from build123d import *

# Parameters (mm, degrees)
SKETCH7_W               = 50.8
SKETCH7_H               = 49.5808
BASE_FLANGE1_DEPTH      = 3
F_10_CLEARANCE_HOLE1_D  = 5
EDGE_FLANGE1_DEPTH      = 50.8
EDGE_FLANGE1_START      = 3
EDGE_FLANGE1_PROFILE_R  = 2.5
EDGE_FLANGE1_FLAT_DEPTH = 3
EDGE_FLANGE2_DEPTH      = 50.8
EDGE_FLANGE2_START      = 3
EDGE_FLANGE2_PROFILE_R  = 2.5
EDGE_FLANGE2_FLAT_DEPTH = 3


# Sheet-metal steps are written as plain solids
with BuildPart() as part:
    # Sketch7 → Base-Flange1 (new body)
    with BuildSketch(Plane(origin=(0, 0, 0), x_dir=(0, -1, 0), z_dir=(-1, 0, 0))):
        with Locations((-25.4, -28.4)):
            Rectangle(SKETCH7_W, SKETCH7_H)
    extrude(amount=-BASE_FLANGE1_DEPTH)

    # #10 Clearance Hole1 (through all)
    with Locations(Plane(origin=(3, 0, 0), x_dir=(0, 0, -1), z_dir=(1, 0, 0))):
        with Locations((41.1, 12.7), (41.1, 25.4), (28.4, 25.4), (28.4, 12.7), (15.7, 12.7), (15.7, 25.4), (15.7, 38.1), (28.4, 38.1), (41.1, 38.1)):
            Hole(F_10_CLEARANCE_HOLE1_D / 2)

    # Edge-Flange1 bend section (across the edge) → Edge-Flange1 (add)
    with BuildSketch(Plane(origin=(3, 0, -53.8), x_dir=(0, 0, 1), z_dir=(0, 1, 0))):
        with BuildLine():
            Line((-3, 0.6096), (0, 0.6096))
            ThreePointArc((0, 0.6096), (0.178547706, 0.178547706), (0.6096, 0))
            Line((0.6096, 0), (0.6096, -3))
            ThreePointArc((0.6096, -3), (-1.942772637, -1.942772637), (-3, 0.6096))
        make_face()
    extrude(amount=EDGE_FLANGE1_DEPTH)

    # Edge-Flange1 profile (on flange) → Edge-Flange1 flat (add)
    with BuildSketch(Plane(origin=(3, 0, -53.8), x_dir=(0, 1, 0), z_dir=(0, 0, -1)).offset(EDGE_FLANGE1_START)):
        Polygon((0, 0.6096), (50.8, 0.6096), (50.8, 3.35), (66.675, 3.35), (73.025, 9.7), (73.025, 47.8), (66.675, 54.15), (50.8, 54.15), (0, 9.7), align=None)
        with Locations((63.5, 9.7)):
            Circle(EDGE_FLANGE1_PROFILE_R, mode=Mode.SUBTRACT)
        with Locations((63.5, 22.4)):
            Circle(EDGE_FLANGE1_PROFILE_R, mode=Mode.SUBTRACT)
        with Locations((63.5, 35.1)):
            Circle(EDGE_FLANGE1_PROFILE_R, mode=Mode.SUBTRACT)
        with Locations((63.5, 47.8)):
            Circle(EDGE_FLANGE1_PROFILE_R, mode=Mode.SUBTRACT)
    extrude(amount=-EDGE_FLANGE1_FLAT_DEPTH)

    # Edge-Flange2 bend section (across the edge) → Edge-Flange2 (add)
    with BuildSketch(Plane(origin=(3, 50.8, -3), x_dir=(0, 0, -1), z_dir=(0, -1, 0))):
        with BuildLine():
            Line((-3, 0.6096), (0, 0.6096))
            ThreePointArc((0, 0.6096), (0.178547706, 0.178547706), (0.6096, 0))
            Line((0.6096, 0), (0.6096, -3))
            ThreePointArc((0.6096, -3), (-1.942772637, -1.942772637), (-3, 0.6096))
        make_face()
    extrude(amount=EDGE_FLANGE2_DEPTH)

    # Edge-Flange2 profile (on flange) → Edge-Flange2 flat (add)
    with BuildSketch(Plane(origin=(3, 0, -3), x_dir=(0, -1, 0), z_dir=(0, 0, 1)).offset(EDGE_FLANGE2_START)):
        Polygon((0, 0.6096), (0, 9.7), (-50.8, 54.15), (-66.675, 54.15), (-73.025, 47.8), (-73.025, 9.7), (-66.675, 3.35), (-50.8, 3.35), (-50.8, 0.6096), align=None)
        with Locations((-63.5, 9.7)):
            Circle(EDGE_FLANGE2_PROFILE_R, mode=Mode.SUBTRACT)
        with Locations((-63.5, 22.4)):
            Circle(EDGE_FLANGE2_PROFILE_R, mode=Mode.SUBTRACT)
        with Locations((-63.5, 35.1)):
            Circle(EDGE_FLANGE2_PROFILE_R, mode=Mode.SUBTRACT)
        with Locations((-63.5, 47.8)):
            Circle(EDGE_FLANGE2_PROFILE_R, mode=Mode.SUBTRACT)
    extrude(amount=-EDGE_FLANGE2_FLAT_DEPTH)


solid = part.part
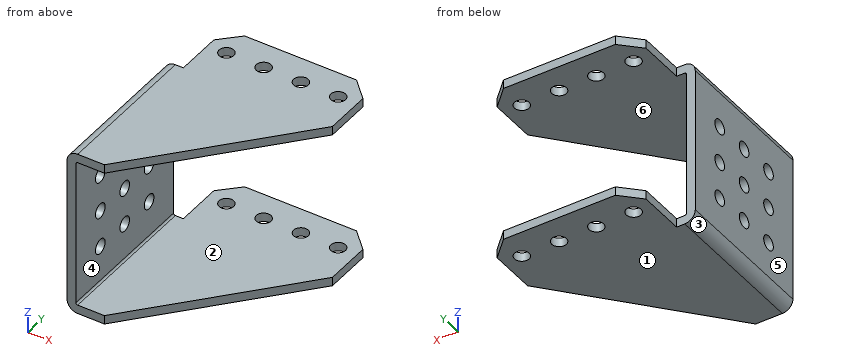
Input: part model. Units: mm. Frame: model coordinates. Face numbers are marked on the shaded views. A direction names the side the tool comes from. Give positions to 0.01 mm unless a question says otherwise; leave off trailing zeros. Order: outer loops, then holes, each group sorted by start corner. A loop starts at its lowest first (then second) coordinate and runs counter-clockwise, first axis right, second up.
Q1. Draft query along Z for the marked faces 3, 4, 5 and 6. Return one class per face: +Z half, -Z half, draft (parallel to the pull), parting line (faces both ways), or undercut.
Checked values:
face 3: -Z half
face 4: undercut
face 5: draft
face 6: undercut
Q2. Set-up query: the marked faces 1 and 2. Return all of +Z, -Z, +X, -X, +Y, -Y with unobstructed straight access to the full face (end or side cutting, diameter ignored); none if empty.
Checked values:
face 1: -Z, +X, -X, +Y, -Y
face 2: +X, +Y, -Y
Q3. Ray query, probe 1 along X at (y, z) = (63.5, -0.9); probe 2 along Y at (x, z) = (1.8, -15.7); probe 3 along Z at (x, y) = (36.5, 31). Return the intervals inside material, ascending.
Checked values:
probe 1: x = 6.35 to 10.2, 15.2 to 22.9, 27.9 to 35.6, 40.6 to 48.3, 53.3 to 57.15
probe 2: y = 0 to 10.2, 15.2 to 22.9, 27.9 to 35.6, 40.6 to 50.8
probe 3: z = -56.8 to -53.8, -3 to 0
Q4. Section D-D on y = 48. Output: boundary loops of the cut face in (x, z), and give its area (3 significant figures).
Checked values:
outline: (0, -53.19) arc R3.61 ccw to (3.61, -56.8) - (54.7, -56.8) - (54.7, -53.8) - (3.61, -53.8) arc R0.61 cw to (3, -53.19) - (3, -3.61) arc R0.61 cw to (3.61, -3) - (54.7, -3) - (54.7, 0) - (3.61, 0) arc R3.61 ccw to (0, -3.61) - close
area: 475 mm2
Q5. Section C-C on x = 38.1. Output: boundary loops of the cut face in (y, z) (3 decimals), and give its area (3 significant figures).
Checked values:
outline: (29.029, -56.8) - (61, -56.8) - (61, -53.8) - (29.029, -53.8) - close; (29.029, -3) - (61, -3) - (61, 0) - (29.029, 0) - close; (66, -56.8) - (73.025, -56.8) - (73.025, -53.8) - (66, -53.8) - close; (66, -3) - (73.025, -3) - (73.025, 0) - (66, 0) - close
area: 234 mm2
Q6. Section A-A on z = -28.4. Output: boundary loops of the cut face in (x, y), and give its area (3 significant figures).
Checked values:
outline: (0, 0) - (3, 0) - (3, 10.2) - (0, 10.2) - close; (0, 15.2) - (3, 15.2) - (3, 22.9) - (0, 22.9) - close; (0, 27.9) - (3, 27.9) - (3, 35.6) - (0, 35.6) - close; (0, 40.6) - (3, 40.6) - (3, 50.8) - (0, 50.8) - close
area: 107 mm2
Q7. Contact query for flat-ended pins moving along their axis: pin 1 Ø6 at (x, z) = (41.5, -50) entering from -Y; pin 2 Ø6.5 at (y, z) = (12.7, -41.1) entering from +X; pin 3 Ø1.5 at (y, z) = (62.5, -1) entering from -X. Output: stop coordinate, or through.
Checked values:
pin 1: passes through
pin 2: stops at x = 3
pin 3: stops at x = 6.35
Q8. Section B-B on y = 12.7. Output: boundary loops of the cut face in (x, z).
Checked values:
outline: (0, -53.19) arc R3.61 ccw to (3.61, -56.8) - (23.81, -56.8) - (23.81, -53.8) - (3.61, -53.8) arc R0.61 cw to (3, -53.19) - (3, -43.6) - (0, -43.6) - close; (0, -38.6) - (3, -38.6) - (3, -30.9) - (0, -30.9) - close; (0, -25.9) - (3, -25.9) - (3, -18.2) - (0, -18.2) - close; (0, -13.2) - (3, -13.2) - (3, -3.61) arc R0.61 cw to (3.61, -3) - (23.81, -3) - (23.81, 0) - (3.61, 0) arc R3.61 ccw to (0, -3.61) - close
